Here's how the part is built. I have some questions about the finished solid (model axes, mm). Coordinates: 2 decimals unless noted, no trailing zeros. Loops run counter-clockwise (first coordinate to the right, second up) from the corner with the lowest first, then second, coordinate; pieces in that order, holes last.
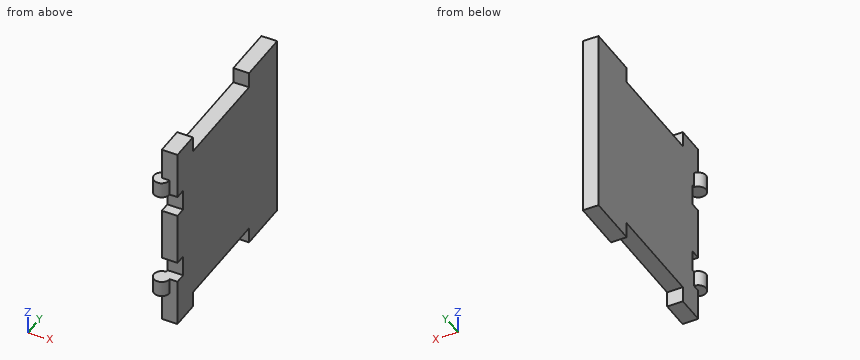
```python
from build123d import *

# Parameters (mm, degrees)
BOSS_EXTRUDE1_DEPTH = 3
SKETCH4_R           = 1.5
BOSS_EXTRUDE2_DEPTH = 3
LPATTERN1_COUNT     = 2
LPATTERN1_PITCH     = 21
SKETCH5_W           = 4
SKETCH5_H           = 2
CUT_EXTRUDE1_DEPTH  = 10


with BuildPart() as part:
    # Sketch1 → Boss-Extrude1 (new body)
    with BuildSketch(Plane(origin=(0, 0, 0), x_dir=(0, 0, -1), z_dir=(1, 0, 0))):
        Polygon((-15, 0), (15, 0), (18, 0), (18, 5.47), (15, 5.47), (15, 25.47), (18, 25.47), (18, 35.47), (15, 35.47), (-15, 35.47), (-18, 35.47), (-18, 25.47), (-15, 25.47), (-15, 5.47), (-18, 5.47), (-18, 0), align=None)
    extrude(amount=BOSS_EXTRUDE1_DEPTH)

    # Sketch4 → Boss-Extrude2 (add)
    with BuildSketch(Plane.XY.offset(12)):
        Circle(SKETCH4_R)
    boss_extrude2 = extrude(amount=-BOSS_EXTRUDE2_DEPTH)

    # LPattern1: Boss-Extrude2 ×2
    with Locations(*[(0, 0, -i * LPATTERN1_PITCH) for i in range(1, LPATTERN1_COUNT)]):
        add(boss_extrude2)

    # Sketch5 → Cut-Extrude1 (cut)
    with BuildSketch(Plane.ZY):
        with Locations((-7, 1)):
            Rectangle(SKETCH5_W, SKETCH5_H)
        with Locations((7, 1)):
            Rectangle(SKETCH5_W, SKETCH5_H)
    extrude(amount=-CUT_EXTRUDE1_DEPTH, mode=Mode.SUBTRACT)


solid = part.part
```
1. I want a section at C-C (z = -3). Please give me the cut outline in (x, y).
2. I want a section at B-B (y = 11.5). Please give me the cut outline in (x, z).
3. I want a section at D-D (x = 0.7). Please give me the cut outline in (y, z), then the cut area to 3 significant figures.
4. I need wall thicknesses on line 1 along X through (y, z) = (25.5, 11); line 2 along Z through (x, y) = (0.1, 10.5); line 3 along Y through (x, z) = (1.85, -1). Which ranges of each line are inside material? Lowest first, please.
5. I want a section at A-A (z = 16). Please give me the cut outline in (x, y), then the cut area to 3 significant figures.
6. For pin 1 (1.5 mm diameter, centred on x = 1, z = -6.5, fed in from -Y); pin 2 (2.5 mm diameter, centred on x = 1, z = 0, fed in from -Y); pin 3 (1.5 mm diameter, centred on x = 2, y = 19, fed in from +Z); pin 4 (1 mm diameter, centred on x = -1, z = -1, fed in from +Y), each with a flat end and sliding along its axis, tell me the tip position at first contact or that it passes through.
Response values:
1. outline: (0, 0) - (3, 0) - (3, 35.47) - (0, 35.47) - close
2. outline: (0, -15) - (3, -15) - (3, 15) - (0, 15) - close
3. outline: (-1.33, -12) - (0, -12) - (0, -18) - (5.47, -18) - (5.47, -15) - (25.47, -15) - (25.47, -18) - (35.47, -18) - (35.47, 18) - (25.47, 18) - (25.47, 15) - (5.47, 15) - (5.47, 18) - (0, 18) - (0, 12) - (-1.33, 12) - (-1.33, 9) - (2, 9) - (2, 5) - (0, 5) - (0, -5) - (2, -5) - (2, -9) - (-1.33, -9) - close
3. area: 1,150 mm2
4. line 1: x = 0 to 3
4. line 2: z = -15 to 15
4. line 3: y = 0 to 35.47
5. outline: (0, 0) - (3, 0) - (3, 5.47) - (0, 5.47) - close; (0, 25.47) - (3, 25.47) - (3, 35.47) - (0, 35.47) - close
5. area: 46.4 mm2
6. pin 1: stops at y = 2
6. pin 2: stops at y = 0
6. pin 3: stops at z = 15
6. pin 4: passes through
